Autodesk Inventor part; units mm, degrees
ref_plane "YZ Plane" through (0, 0, 0) normal (1, 0, 0) x (0, 1, 0)
ref_plane "XZ Plane" through (0, 0, 0) normal (0, 1, 0) x (-1, 0, 0)
ref_plane "XY Plane" through (0, 0, 0) normal (0, 0, 1) x (1, 0, 0)
sketch "Boceto1" plane through (0, 0, 0) normal (0, 0, 1) x (1, 0, 0)
  line L0 (-76, 6) -> (76, 6)
  line L1 (76, 6) -> (76, -6)
  line L2 (76, -6) -> (-76, -6)
  line L3 (-76, -6) -> (-76, 6)
  circle A0 centre (0, 0) radius 1.5
  circle A1 centre (57, 0) radius 1.5
  circle A2 centre (-57, 0) radius 1.5
  circle A3 centre (-9.5, 0) radius 0.65
  circle A4 centre (9.5, 0) radius 0.65
  circle A5 centre (28.5, 0) radius 0.65
  circle A6 centre (47.5, 0) radius 0.65
  circle A7 centre (66.5, 0) radius 0.65
  circle A8 centre (-28.5, 0) radius 0.65
  circle A9 centre (-47.5, 0) radius 0.65
  circle A10 centre (-66.5, 0) radius 0.65
  point P0 (-76, 0)
  point P1 (0, 6)
  dimension "d0" = 152
  dimension "d1" = 12
  dimension "d2" = 3
  dimension "d3" = 3
  dimension "d4" = 3
  dimension "d5" = 57
  dimension "d6" = 57
  dimension "d7" = 1.3
  dimension "d8" = 1.3
  dimension "d9" = 19
  dimension "d10" = 9.5
  dimension "d13" = 19
  dimension "d20" = 19
extrude "Extrusión1" add sketch "Boceto1" along normal blind 12
sketch "Boceto2" plane through (0, 0, 12) normal (0, 0, 1) x (1, 0, 0)
  circle A0 centre (-66.5, 0) radius 0.65
  circle A1 centre (-66.5, 0) radius 2.5
  line L0 (-76, 0) -> (76, 0) construction
  line L1 (76, -6) -> (76, 6) construction
  circle A2 centre (-47.5, 0) radius 2.5
  circle A3 centre (-28.5, 0) radius 2.5
  circle A4 centre (-9.5, 0) radius 2.5
  circle A5 centre (9.5, 0) radius 2.5
  circle A6 centre (28.5, 0) radius 2.5
  circle A7 centre (47.5, 0) radius 2.5
  circle A8 centre (66.5, 0) radius 2.5
  point P0 (0, 0)
  dimension "d27" = 5
  dimension "d30" = 19
  dimension "d35" = 152
extrude "Extrusión2" cut sketch "Boceto2" against normal blind 1.5 contours A0 | A1 | A2 | A3 | A4 | A5 | A6 | A7 | A8
fillet "Empalme1" radius 2 4 edges at (-76, -6, 6) (76, -6, 6) (76, 6, 6) (-76, 6, 6)
equation "\"d8\" = d7"
properties part number "Guia fibra 8Ch V2_2"
Input: part model. Units: mm. Frame: model coordinates. A direction names the side the tool comes from. Give positions to 0.01 mm unless a question says otherwise; leave off trailing zeros. Order: outer loops, then holes, each group sorted by start corner. A loop starts at its lowest first (then second) coordinate and runs counter-clockwise, first axis right, second up.
1. Material intervals for L1, parallel to Y at x = 57, z = 3; L2, parallel to X at y = 1, z = 6.5; L3, parallel to Y at x = -9.5, z = 6, sorted ascending.
Derived:
L1: y = -6 to -1.5, 1.5 to 6
L2: x = -76 to -58.12, -55.88 to -1.12, 1.12 to 55.88, 58.12 to 76
L3: y = -6 to -0.65, 0.65 to 6
2. Section B-B on z = 1.25. Give the number of separate pieces and of enclosed holes in the cut face, and give its area (3 significant figures).
Derived:
separate pieces: 1
enclosed holes: 11
area: 1,790 mm2
3. Pin query (flat end, axial travel): pin 1 (1.5 mm diameter, centred on x = -67.5, y = 0, fed in from +Z). Return the tip coordinate at first contact, or that it passes through.
Derived:
pin 1: stops at z = 10.5
4. Section A-A on x = -57. Return the cut outline in (y, z).
Derived:
outline: (-6, 0) - (-1.5, 0) - (-1.5, 12) - (-6, 12) - close; (1.5, 0) - (6, 0) - (6, 12) - (1.5, 12) - close
5. Mould query, pull axis Y, two halves, no side actions, for faces 3 (the flat face through (1, -6, 6)), 4 (the flat face through (-76, 0, 6)), 5 (the cylindrical face through (-31, 0, 11)). Classes: released by +Y, released by -Y, zero draft, split by the parting line, or undercut.
Derived:
face 3: released by -Y
face 4: zero draft
face 5: undercut
6. Reachability of faces 1 (the flat face through (67, -1, 10.5)), 2 (the cylindrical face through (-55.57, -0.45, 5.92)) from +Z, -Z, +X, -X, +Y, -Y: full face, straight path, thin tool, end or side. Return the list, or none.
Derived:
face 1: +Z
face 2: +Z, -Z
